Here's how the part is built. I have some questions about the finished solid (model axes, mm). A direction names the side the tool comes from. Round coordinates to 2 decimals unless told otherwise and drop trailing zeros. Order: outer loops, then holes, each group sorted by start corner. A loop starts at its lowest first (then second) coordinate and runs counter-clockwise, first axis right, second up. Notation, with made-up numbers: M 75.5,-29 L 128.5,-29 A35 cw 128.5,9 Z; hole C -22,42 d2. An arc over 180 degrees is marked long. Write item = value, one per line. Start each with the question number.
Item 1: For faces 1 (the face through (-25, -14, -10.5)), 2 (the face through (-5.82, 48.52, -10.75)), 3 (the face through (-7.25, 48, 0)), 4 (the face through (0, -37, 12.5)), which set-ups out of +Z, -Z, +X, -X, +Y, -Y let a thin tool reach every point of the face, with its end or its side?
Item 2: I want a section at A-A, the plane z = 0. List the corners of the cut face in (x, y) for me.
Item 3: Please list where these lines run through material, in increasing order: L1, parallel to Z at x = 0, y = 38.5; L2, parallel to Z at x = 0, y = 48.25; L3, parallel to X at y = 0, z = -12.1.
Item 4: We'd pull the mould along Y, two halves only. Please class faces 5 (the face through (26.327, 10.916, 3.979)), 6 (the face through (-9.43, 42.466, 0.203)), 7 (the face through (30.493, 0.671, 7.965)), 8 (the face through (7.5, -37, 0)): pulls with the +Y half, pulls with the -Y half, needs draft (parallel to the pull), parting line crosses it, or undercut.
Item 5: I want a section at D-D, the plane x = -38. List the corners of the cut face in (y, z) for me.
Item 6: I'm going to push flat-ended pins straight in: P1, Ø10, axis at x = -31.5, z = 10.5, coming from the -Y side; P2, Ø2, axis at y = -15.5, z = -8.5, coming from the +X side; P3, Ø2, axis at y = 37.5, z = 9.5, coming from the -X side; P4, Ø18.5, axis at x = 10.5, y = 0.5, coming from the -Z side. Where does each tip first touch, or does it pass through?
```python
from build123d import *

# Parameters (mm, degrees)
F3_W     = 15
F3_H     = 25
F4_DEPTH = 12.5
F6_W     = 14.5
F6_H     = 24.5
F7_DEPTH = 14
F8_D     = 5
F9_R     = 5


with BuildPart() as f1:
    # F0 (on Front) → F1 (revolve)
    with BuildSketch(Plane.XZ):
        Polygon((43.5, 14.5), (28.5, 14.5), (28.5, 10.5), (30.5, 10.5), (30.5, 5.5), (28.5, 5.5), (28.5, 2.5), (30.5, 2.5), (30.5, -2.5), (28.5, -2.5), (28.5, -5.5), (30.5, -5.5), (30.5, -10.5), (28.5, -10.5), (28.5, -14.5), (43.5, -14.5), align=None)
    revolve(axis=Axis((0, 0, 1.261241), (0, 0, -1)))

    # F3 (on offset) → F4 (cut)
    with BuildSketch(Plane.XZ.offset(43.5)):
        Rectangle(F3_W, F3_H)
    extrude(amount=-F4_DEPTH, mode=Mode.SUBTRACT)

    # F6 (on offset) → F7 (join)
    with BuildSketch(Plane.XZ.offset(-40)):
        Rectangle(F6_W, F6_H)
    extrude(amount=-F7_DEPTH)

    # F8 (through all)
    with Locations(Plane.XZ.offset(43.5)):
        with Locations((0, 8), (0, 0), (0, -8)):
            Hole(F8_D / 2)

    # F9
    f9_edges = [f1.edges().sort_by_distance(p)[0] for p in [
        (-7.5, -36.924285, 12.5),
        (7.5, -36.924285, 12.5),
        (-7.5, -36.924285, -12.5),
        (7.5, -36.924285, -12.5),
        (7.25, 48.445789, 12.25),
        (-7.25, 48.445789, 12.25),
        (7.25, 48.445789, -12.25),
        (-7.25, 48.445789, -12.25),
    ]]
    fillet(f9_edges, radius=F9_R)


solid = f1.part
```
Filled in:
q1.face_1 = none
q1.face_2 = -Z, -X, +Y
q1.face_3 = +Z, -Z, -X, +Y
q1.face_4 = -Y
q2.outline = M -7.5,-42.85 L -7.5,-31 L -2.5,-31 L -2.5,-30.4 A30.5 cw -2.5,30.4 L -2.5,54 L -7.25,54 L -7.25,42.89 A43.5 ccw Z; M 2.5,-31 L 7.5,-31 L 7.5,-42.85 A43.5 ccw 7.25,42.89 L 7.25,54 L 2.5,54 L 2.5,30.4 A30.5 cw 2.5,-30.4 Z
q3.L1 = -14.5 to -10.5, -5.5 to -2.5, 2.5 to 5.5, 10.5 to 14.5
q3.L2 = -12.25 to -10.5, -5.5 to -2.5, 2.5 to 5.5, 10.5 to 12.25
q3.L3 = -43.5 to -28.5, 28.5 to 43.5
q4.face_5 = undercut
q4.face_6 = parting line crosses it
q4.face_7 = undercut
q4.face_8 = needs draft
q5.outline = M -21.17,-14.5 L 21.17,-14.5 L 21.17,14.5 L -21.17,14.5 Z
q6.P1 = -34.5
q6.P2 = 41.01
q6.P3 = -23.66
q6.P4 = through
